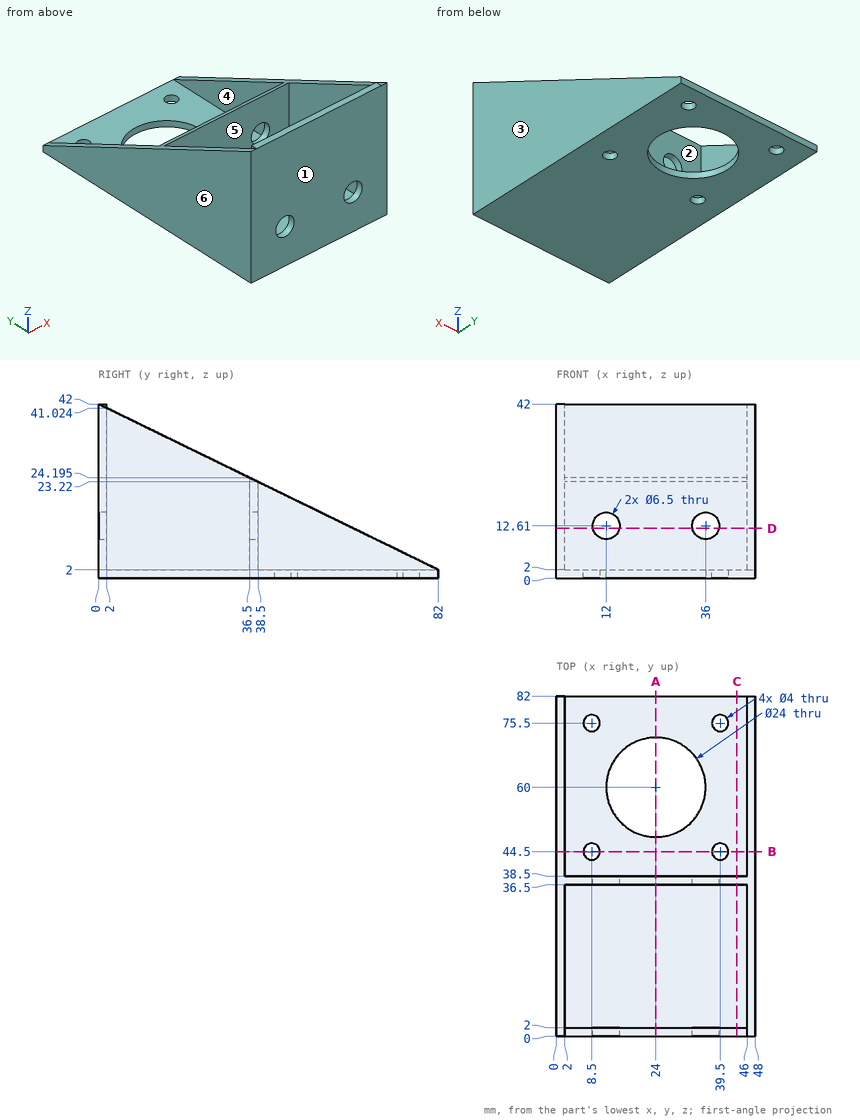
For this review, use the dimensioned drawing (mm, ordinates from the lowest corner) and the shaded views. A direction names the side the tool comes from. Round coordinates to 2 decimals unless told otherwise and drop trailing zeros. Write each loop counter-clockwise with the first axis right and the second up, starting at its lowest first coordinate (ties: lowest second). Pieces come first, ordered by that corner, then holes. Notation, with made-up numbers: (6, 71) - (25, 71) arc R26 ccw to (25, 95) - close; hole circle Ø6 at (56.25, 23.25). An arc over 180 degrees is marked (long way). One line per item, written item: value. Start each with the question number.
1. To check wall thickness, follow L1, parallel to Y at x = 21, z = 5; L2, parallel to X at y = 65, z = 2.5; L3, parallel to Z at x = 44.5, y = 45. State the ranges of each line that lie inside material, in increasing order. Write a range as from..to.
2. Consider section A-A on x = 24. Write out the cut boundary in (y, z) (1 decimal).
3. Consider section C-C on x = 43.5. Write out the cut boundary in (y, z) (1 decimal).
4. Clearance check with flat-ended pins moving along their axes: P1, Ø7.5, axis at x = 36, z = 12.61, coming from the +Y side; P2, Ø4, axis at x = 17.5, y = 46, coming from the +Z side. State where each tip first meets the part, or that it passes through.
5. The part is to be moulded in two halves that separate along X. For the marked faces 1, 2 and 3, say which applies: released by +X, released by -X, zero draft, split by the parting line, or undercut.
6. Machinability: for the marked faces 4, 5 and 6, which of the approach directions +Z, -Z, +X, -X, +Y, -Y give a long, thin tool a straight path to every point of the face, cutting with its end or side? Answer none if there is none.
7. Consider section D-D on z = 12. Write out the cut boundary in (x, y), and give its area (3 significant figures).
8. Consider section B-B on y = 44.5. Write out the cut boundary in (x, z), and give its area (3 significant figures).
Checks:
1. L1: y = 0..2, 36.5..38.5
1. L2: x = 0..2, 46..48
1. L3: z = 0..2
2. outline: (0, 0) - (48, 0) - (48, 2) - (38.5, 2) - (38.5, 23.2) - (36.5, 24.2) - (36.5, 2) - (2, 2) - (2, 42) - (0, 42) - close; (72, 0) - (82, 0) - (82, 2) - (72, 2) - close
3. outline: (0, 0) - (82, 0) - (82, 2) - (38.5, 2) - (38.5, 23.2) - (36.5, 24.2) - (36.5, 2) - (2, 2) - (2, 42) - (0, 42) - close
4. P1: stops at y = 38.5
4. P2: stops at z = 2
5. face 1: zero draft
5. face 2: undercut
5. face 3: released by +X
6. face 4: +Z, +Y
6. face 5: +Z
6. face 6: +Z, -Z, -X, +Y, -Y
7. outline: (0, 0) - (8.81, 0) - (8.81, 2) - (2, 2) - (2, 36.5) - (8.81, 36.5) - (8.81, 38.5) - (2, 38.5) - (2, 61.5) - (0, 61.5) - close; (15.19, 0) - (32.81, 0) - (32.81, 2) - (15.19, 2) - close; (15.19, 36.5) - (32.81, 36.5) - (32.81, 38.5) - (15.19, 38.5) - close; (39.19, 0) - (48, 0) - (48, 61.5) - (46, 61.5) - (46, 38.5) - (39.19, 38.5) - (39.19, 36.5) - (46, 36.5) - (46, 2) - (39.19, 2) - close
7. area: 371 mm^2
8. outline: (0, 0) - (6.5, 0) - (6.5, 2) - (2, 2) - (2, 20.29) - (0, 20.29) - close; (10.5, 0) - (37.5, 0) - (37.5, 2) - (10.5, 2) - close; (41.5, 0) - (48, 0) - (48, 20.29) - (46, 20.29) - (46, 2) - (41.5, 2) - close
8. area: 153 mm^2
